Source: three-view drawing plus pictorial views. Frame: mm from the lowest corner of the part. A direction names the side the tool comes from. Coordinates: 2 decimals unless noted, no trailing zeros. Loops run counter-clockwise (first coordinate to the right, second up) from the corner with the lowest first, then second, coordinate; pieces in that order, holes last. Notation, with made-up numbers: (26.5, 21) - (75.5, 21) arc R14 ccw to (75.5, 31) - close; hole circle Ø6 at (31, 33.25). An arc over 180 degrees is marked (long way). Return JSON: item names as keys, results as strings.
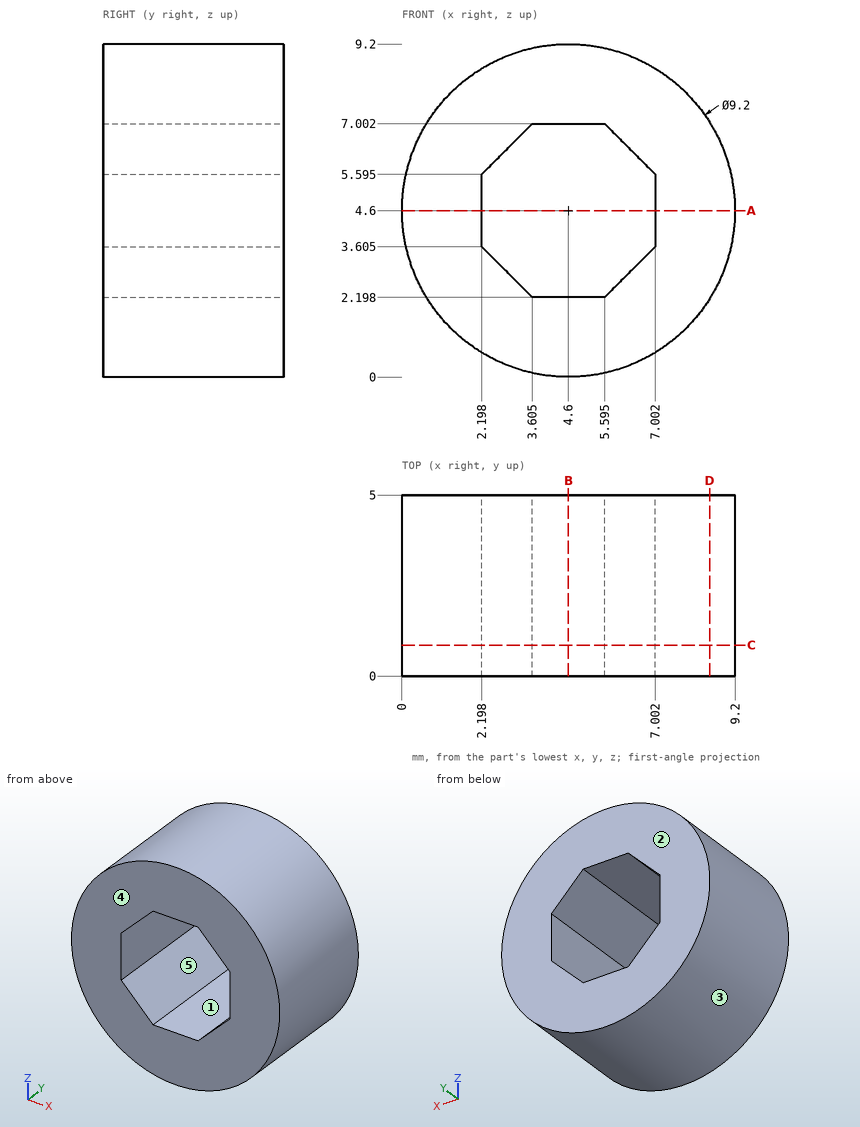
Item 1: Section query D-D, the plane x = 8.5. Return loops of the section in (y, z).
Worked out:
{"outline": "(0, 2.16) - (5, 2.16) - (5, 7.04) - (0, 7.04) - close"}
Item 2: Mould query, pull axis Z, two halves, no side actions, for the marked faces 3, 4 and 5. Classes: +Z half, -Z half, draft (parallel to the pull), parting line (faces both ways), or undercut.
Worked out:
{"face 3": "parting line", "face 4": "draft", "face 5": "undercut"}
Item 3: Section query A-A, the plane z = 4.6. Return loops of the section in (x, y), and give its area (3 significant figures).
Worked out:
{"outline": "(0, 0) - (2.2, 0) - (2.2, 5) - (0, 5) - close; (7, 0) - (9.2, 0) - (9.2, 5) - (7, 5) - close", "area": "22.0 mm^2"}
Item 4: Reachability of the marked faces 1 and 2 from +Z, -Z, +X, -X, +Y, -Y: full face, straight path, thin tool, end or side. Return the list, or none.
Worked out:
{"face 1": "+Y, -Y", "face 2": "+Z, -Z, +X, -X, +Y"}
Item 5: Section query C-C, the plane y = 0.85. Return loops of the section in (x, z) (3 decimals).
Worked out:
{"outline": "circle Ø9.2 at (4.6, 4.6); hole (2.198, 3.605) - (3.605, 2.198) - (5.595, 2.198) - (7.002, 3.605) - (7.002, 5.595) - (5.595, 7.002) - (3.605, 7.002) - (2.198, 5.595) - close"}
Item 6: Section query B-B, the plane x = 4.6. Return loops of the section in (y, z).
Worked out:
{"outline": "(0, 0) - (5, 0) - (5, 2.2) - (0, 2.2) - close; (0, 7) - (5, 7) - (5, 9.2) - (0, 9.2) - close"}
Item 7: Ray query, probe 1 along Z at (x, y) = (5.25, 1.75); probe 2 along Z at (x, y) = (3.5, 4.6); probe 3 along X at (y, z) = (4.8, 3.25). Return the intervals inside material, ascending. Write a range as from..to.
Worked out:
{"probe 1": "0.05..2.2, 7..9.15", "probe 2": "0.13..2.3, 6.9..9.07", "probe 3": "0.2..2.55, 6.65..9"}
Item 8: First-contact query: pin 1 Ø1 at (x, z) = (2.5, 7.5) entering from -Y; pin 2 Ø1.5 at (x, y) = (7, 4.5) entering from -Z; pin 3 Ø1 at (x, z) = (5.5, 5.5) entering from -Y. Flat tips, straight axial feed; report the tip coordinate or a pass-through.
Worked out:
{"pin 1": "y = 0", "pin 2": "z = 0.31", "pin 3": "through"}
